Here's how the part is built. I have some questions about the finished solid (model axes, mm). Face numbers are marked on the shaded views. Round coordinates to 2 decimals unless told otherwise and drop trailing zeros. Order: outer loops, then holes, each group sorted by start corner. A loop starts at its lowest first (then second) coordinate and runs counter-clockwise, first axis right, second up. Notation, with made-up numbers: (71.25, -5.5) -> (98.25, -5.5) arc R20 ccw to (98.25, 16.5) -> close; hole circle Ø9 at (-39.5, -19.5). An arc over 180 degrees is marked (long way). One line per item, written item: value.
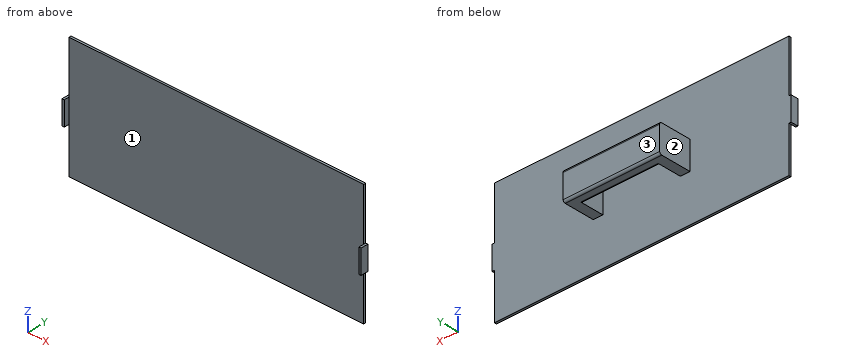
```python
from build123d import *

# Parameters (mm, degrees)
BOSS_EXTRUDE1_DEPTH = 1
SKETCH3_W           = 4.432871169
SKETCH3_H           = 12.941954118
SKETCH3_W_2         = 4.432871168
BOSS_EXTRUDE4_DEPTH = 10
SKETCH4_W           = 44.535219178
SKETCH4_H           = 12.941954118
BOSS_EXTRUDE6_DEPTH = 5
FILLET3_R           = 1
FILLET4_R           = 1
SKETCH7_W           = 10.96861972
SKETCH7_H           = 3.370404632
BOSS_EXTRUDE7_DEPTH = 1
SKETCH9_W           = 10.96861972
SKETCH9_H           = 3.370404632
BOSS_EXTRUDE8_DEPTH = 1


with BuildPart() as part:
    # Sketch1 → Boss-Extrude1 (new body)
    with BuildSketch(Plane(origin=(0, 0, 0), x_dir=(1, 0, 0), z_dir=(0, 1, 0))):
        Polygon((76.937608383, -62.782038713), (76.937608383, -8.810873689), (-58.911197585, -8.810873689), (-58.911197585, -62.792119939), (-58.911197585, -64.768415651), (-56.350218844, -64.768415651), (74.598736982, -64.768415651), (76.937608383, -64.768415651), align=None)
    extrude(amount=BOSS_EXTRUDE1_DEPTH)

    # Sketch3 → Boss-Extrude4 (add)
    with BuildSketch(Plane(origin=(0, 1, 0), x_dir=(1, 0, 0), z_dir=(0, 1, 0))):
        with Locations((-11.037968606, -36.78964467)):
            Rectangle(SKETCH3_W, SKETCH3_H)
        with Locations((29.064379404, -36.78964467)):
            Rectangle(SKETCH3_W_2, SKETCH3_H)
    extrude(amount=BOSS_EXTRUDE4_DEPTH)

    # Sketch4 → Boss-Extrude6 (add)
    with BuildSketch(Plane(origin=(0, 11, 0), x_dir=(1, 0, 0), z_dir=(0, 1, 0))):
        with Locations((9.013205399, -36.78964467)):
            Rectangle(SKETCH4_W, SKETCH4_H)
    extrude(amount=BOSS_EXTRUDE6_DEPTH)

    # Fillet3
    fillet3_edges = [part.edges().sort_by_distance(p)[0] for p in [
        (9.013205399, 16, 30.318667611),
        (9.013205399, 16, 43.260621729),
    ]]
    fillet(fillet3_edges, radius=FILLET3_R)

    # Fillet4
    fillet4_edges = [part.edges().sort_by_distance(p)[0] for p in [
        (9.013205399, 11, 43.260621729),
        (9.013205399, 11, 30.318667611),
    ]]
    fillet(fillet4_edges, radius=FILLET4_R)

    # Sketch7 → Boss-Extrude7 (add)
    with BuildSketch(Plane.ZY.offset(58.911197585)):
        with Locations((35.300658133, -0.685202316)):
            Rectangle(SKETCH7_W, SKETCH7_H)
    extrude(amount=BOSS_EXTRUDE7_DEPTH)

    # Sketch9 → Boss-Extrude8 (add)
    with BuildSketch(Plane(origin=(76.937608383, 0, 0), x_dir=(0, 0, -1), z_dir=(1, 0, 0))):
        with Locations((-35.300658133, -0.685202316)):
            Rectangle(SKETCH9_W, SKETCH9_H)
    extrude(amount=BOSS_EXTRUDE8_DEPTH)


solid = part.part
```
Q1. I want a section at D-D on z = 15. Write out the boundary of the cut face in (x, y), then the cut area to 3 significant figures.
Answers:
outline: (-58.91, 0) -> (76.94, 0) -> (76.94, 1) -> (-58.91, 1) -> close
area: 136 mm2
Q2. For P1, Ø11, axis at x = 4, y = 9, coming from the -Z side; P2, Ø12, axis at x = -44.5, z = 23, coming from the -Y side; P3, Ø0.5, axis at x = 77.5, y = -0.5, coming from the +Z side, each with a flat end and sliding along its axis, tell me the tip position at first contact or that it passes through.
Answers:
P1: z = 30.32
P2: y = 0
P3: z = 40.78
Q3. I want a section at A-A on y = 9.25. Write out the boundary of the cut face in (x, z).
Answers:
outline: (-13.25, 30.32) -> (-8.82, 30.32) -> (-8.82, 43.26) -> (-13.25, 43.26) -> close; (26.85, 30.32) -> (31.28, 30.32) -> (31.28, 43.26) -> (26.85, 43.26) -> close
Q4. If we mould it in two halves opening along X, with no side actions, what happens to the marked faces 1, 2 and 3? For each: pulls with the +X half, pulls with the -X half, needs draft (parallel to the pull), parting line crosses it, or undercut.
Answers:
face 1: undercut
face 2: pulls with the -X half
face 3: needs draft
Q5. I want a section at B-B on z = 35.5. Write out the boundary of the cut face in (x, y).
Answers:
outline: (-59.91, -2.37) -> (-58.91, -2.37) -> (-58.91, 0) -> (76.94, 0) -> (76.94, -2.37) -> (77.94, -2.37) -> (77.94, 1) -> (31.28, 1) -> (31.28, 16) -> (-13.25, 16) -> (-13.25, 1) -> (-59.91, 1) -> close; hole (-8.82, 1) -> (26.85, 1) -> (26.85, 11) -> (-8.82, 11) -> close
Q6. I want a section at C-C on x = 30. Write out the boundary of the cut face in (y, z), then the cut area to 3 significant figures.
Answers:
outline: (0, 8.81) -> (1, 8.81) -> (1, 30.32) -> (15, 30.32) arc R1 ccw to (16, 31.32) -> (16, 42.26) arc R1 ccw to (15, 43.26) -> (1, 43.26) -> (1, 64.77) -> (0, 64.77) -> close
area: 250 mm2
Q7. I need wall thicknesses on line 1 along X through (y, z) = (-0.25, 39.5); line 2 along Y through (x, z) = (8, 36.5); line 3 along Y through (x, z) = (3.5, 16). Which ranges of each line are inside material? Lowest first, please.
Answers:
line 1: -59.91 to -58.91, 76.94 to 77.94
line 2: 0 to 1, 11 to 16
line 3: 0 to 1
